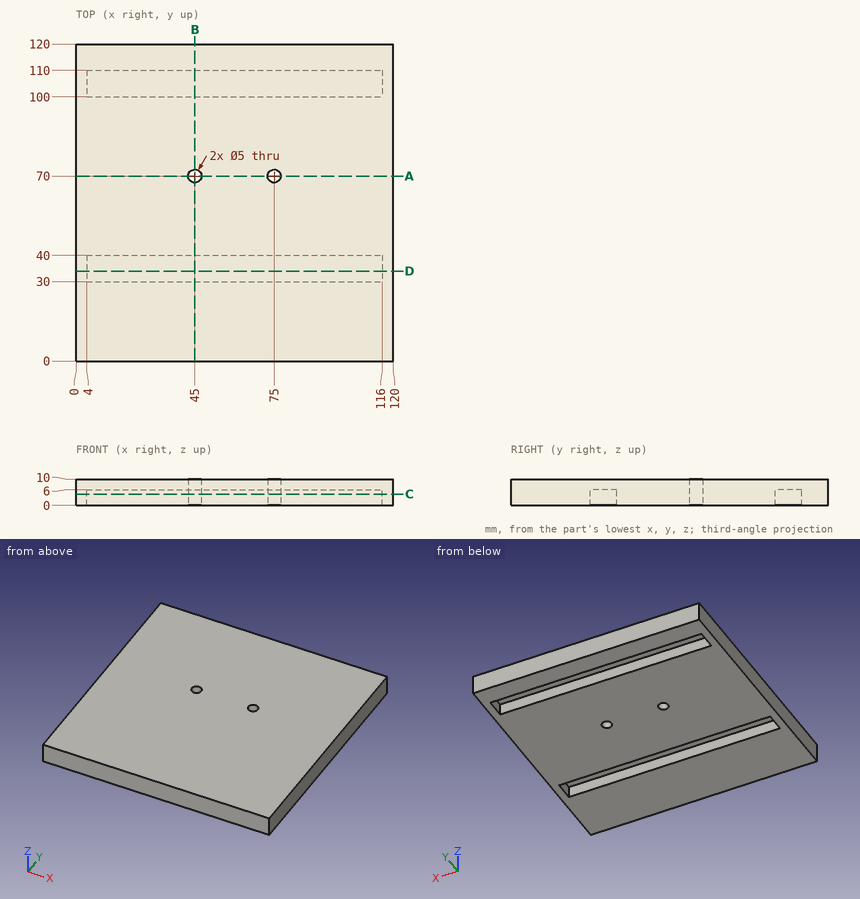
Geometry check sheet. Reference: drawing and pictorial views, mm from the part's lowest x, y, z. Coordinates: 2 decimals unless noted, no trailing zeros. Order: outer loops, then holes, each group sorted by start corner. A loop starts at its lowest first (then second) coordinate and runs counter-clockwise, first axis right, second up.
Item 1: Section check C-C (z = 4.25). Enter the section's corners in (x, y), plus the area to 3 significant figures.
Item 2: Depth check by flat-ended pin: pin 1 (5 mm diameter, centred on x = 36, y = 107, fed in from -Z). Enter the tip coordinate at first touch or a pass-through.
Item 3: Scan lines: line 1 along Y through (x, z) = (70, 1); line 2 along Y through (x, z) = (75, 5.25); line 3 along X through (y, z) = (103.5, 5.5). Record each from-to range of solid material in increasing order.
Item 4: Section check D-D (y = 34). Enter the section's corners in (x, z).
Item 5: Section check A-A (y = 70). Enter the section's corners in (x, z).
Item 6: Section check B-B (x = 45). Enter the section's corners in (y, z).
Check sheet entries:
1. outline: (0, 0) - (120, 0) - (120, 120) - (0, 120) - close; hole (4, 30) - (116, 30) - (116, 40) - (4, 40) - close; hole (4, 100) - (116, 100) - (116, 110) - (4, 110) - close; hole circle Ø5 at (45, 70); hole circle Ø5 at (75, 70)
1. area: 12,100 mm2
2. pin 1: stops at z = 6
3. line 1: y = 0 to 30, 40 to 100, 110 to 120
3. line 2: y = 0 to 30, 40 to 67.5, 72.5 to 100, 110 to 120
3. line 3: x = 0 to 4, 116 to 120
4. outline: (0, 0) - (4, 0) - (4, 6) - (116, 6) - (116, 0) - (120, 0) - (120, 10) - (0, 10) - close
5. outline: (0, 0) - (42.5, 0) - (42.5, 10) - (0, 10) - close; (47.5, 0) - (72.5, 0) - (72.5, 10) - (47.5, 10) - close; (77.5, 0) - (120, 0) - (120, 10) - (77.5, 10) - close
6. outline: (0, 0) - (30, 0) - (30, 6) - (40, 6) - (40, 0) - (67.5, 0) - (67.5, 10) - (0, 10) - close; (72.5, 0) - (100, 0) - (100, 6) - (110, 6) - (110, 0) - (120, 0) - (120, 10) - (72.5, 10) - close
